from build123d import *

# Parameters (mm, degrees)
SKETCH1_W           = 26
SKETCH1_H           = 50
BOSS_EXTRUDE1_DEPTH = 8
SKETCH2_W           = 26
SKETCH2_H           = 50
BOSS_EXTRUDE2_DEPTH = 8
SKETCH3_W           = 26
SKETCH3_H           = 7
BOSS_EXTRUDE3_DEPTH = 36
SKETCH4_R           = 8
SKETCH4_R_2         = 5
BOSS_EXTRUDE4_DEPTH = 10
FILLET2_R           = 3
SKETCH6_W           = 7
SKETCH6_H           = 17
BOSS_EXTRUDE5_DEPTH = 20
CHAMFER1_SIZE       = 2
CUT_EXTRUDE2_DEPTH  = 0.5
CUT_EXTRUDE3_DEPTH  = 0.5
CUT_EXTRUDE4_REACH  = 90.986
SKETCH11_W          = 26
SKETCH11_H          = 10
CUT_EXTRUDE5_DEPTH  = 3
SKETCH12_W          = 26
SKETCH12_H          = 10
CUT_EXTRUDE6_DEPTH  = 3
CUT_EXTRUDE7_REACH  = 90.986
SKETCH13_R          = 1.5
SKETCH14_W          = 39.670907723
SKETCH14_H          = 70.738486061
CUT_EXTRUDE8_DEPTH  = 8
SKETCH15_W          = 26
SKETCH15_H          = 39.127202372
CUT_EXTRUDE9_DEPTH  = 28.5


with BuildPart() as part:
    # Sketch1 → Boss-Extrude1 (new body)
    with BuildSketch(Plane.XY):
        with Locations((37.264100782, -29)):
            Rectangle(SKETCH1_W, SKETCH1_H)
        with BuildLine():
            Line((39.049457889, -22.265997948), (35.478743675, -22.265997948))
            ThreePointArc((35.478743675, -22.265997948), (34.764100782, -20.515997948), (35.478743675, -18.765997947))
            Line((35.478743675, -18.765997947), (39.049457889, -18.765997947))
            ThreePointArc((39.049457889, -18.765997947), (39.764100782, -20.515997948), (39.049457889, -22.265997948))
        make_face(mode=Mode.SUBTRACT)
    extrude(amount=BOSS_EXTRUDE1_DEPTH)



with BuildPart() as body_2:
    # Sketch2 → Boss-Extrude2 (new body)
    with BuildSketch(Plane(origin=(0, 0, -20), x_dir=(-1, 0, 0), z_dir=(0, 0, -1))):
        with Locations((-37.264100782, -29)):
            Rectangle(SKETCH2_W, SKETCH2_H)
        with BuildLine():
            Line((-39.049457889, -18.765997947), (-35.478743675, -18.765997947))
            ThreePointArc((-35.478743675, -18.765997947), (-34.764100782, -20.515997948), (-35.478743675, -22.265997948))
            Line((-35.478743675, -22.265997948), (-39.049457889, -22.265997948))
            ThreePointArc((-39.049457889, -22.265997948), (-39.764100782, -20.515997948), (-39.049457889, -18.765997947))
        make_face(mode=Mode.SUBTRACT)
    extrude(amount=BOSS_EXTRUDE2_DEPTH)


with BuildPart() as part_1:
    add(part.part)

    add(body_2.part)  # Boss-Extrude3 merges body 2
    # Sketch3 → Boss-Extrude3 (add)
    with BuildSketch(Plane.XY.offset(8)):
        with Locations((37.264100782, -50.5)):
            Rectangle(SKETCH3_W, SKETCH3_H)
    extrude(amount=-BOSS_EXTRUDE3_DEPTH)

    # Sketch4 → Boss-Extrude4 (add)
    with BuildSketch(Plane.XZ.offset(54)):
        with Locations(Location((37.264100782, -10, 0), (0, 0, 90))):
            Circle(SKETCH4_R)
        with Locations(Location((37.264100782, -10, 0), (0, 0, 270))):
            Circle(SKETCH4_R_2, mode=Mode.SUBTRACT)
    extrude(amount=BOSS_EXTRUDE4_DEPTH)

    # Fillet2
    fillet2_edges = [part_1.edges().sort_by_distance(p)[0] for p in [
        (24.264100782, -29, 8),
        (24.264100782, -29, -28),
    ]]
    fillet(fillet2_edges, radius=FILLET2_R)

    # Sketch6 → Boss-Extrude5 (add)
    with BuildSketch(Plane.XY.offset(-20)):
        with Locations((27.764100782, -45.5)):
            Rectangle(SKETCH6_W, SKETCH6_H)
    extrude(amount=BOSS_EXTRUDE5_DEPTH)

    # Chamfer1
    chamfer1_edges = [part_1.edges().sort_by_distance(p)[0] for p in [
        (37.264100782, -54, -18),
    ]]
    chamfer(chamfer1_edges, length=CHAMFER1_SIZE)

    # Sketch7 → Cut-Extrude2 (cut)
    with BuildSketch(Plane(origin=(0, 0, 0), x_dir=(-1, 0, 0), z_dir=(0, 0, -1))):
        Polygon((-50.264100782, -4), (-50.264100782, -47), (-31.264100782, -47), (-31.264100782, -37), (-24.264100782, -37), (-24.264100782, -4), align=None)
    extrude(amount=-CUT_EXTRUDE2_DEPTH, mode=Mode.SUBTRACT)

    # Sketch8 → Cut-Extrude3 (cut)
    with BuildSketch(Plane.XY.offset(-20)):
        Polygon((50.264100782, -47), (50.264100782, -4), (24.264100782, -4), (24.264100782, -37), (31.264100782, -37), (31.264100782, -47), align=None)
    extrude(amount=-CUT_EXTRUDE3_DEPTH, mode=Mode.SUBTRACT)

    # Cut-Extrude4: up to this face of the body (flat: up to its plane)
    cut_extrude4_end = Plane(part_1.part.faces().sort_by_distance((38.785185957, -29.119257779, -28))[0])
    # Sketch10 → Cut-Extrude4 (cut, up to the picked face)
    with BuildSketch(Plane.XY.offset(8), mode=Mode.PRIVATE) as cut_extrude4_sk1:
        with BuildLine():
            Line((50.264100782, -20.515997948), (50.264100782, 2.26582648))
            Line((50.264100782, 2.26582648), (24.264100782, 2.26582648))
            Line((24.264100782, 2.26582648), (24.264100782, -20.515997948))
            ThreePointArc((24.264100782, -20.515997948), (37.264100782, -7.515997948), (50.264100782, -20.515997948))
        make_face()
    cut_extrude4_tool1 = split(extrude(cut_extrude4_sk1.sketch, amount=-CUT_EXTRUDE4_REACH, mode=Mode.PRIVATE), bisect_by=cut_extrude4_end, keep=Keep.BOTH, mode=Mode.PRIVATE)
    add(cut_extrude4_tool1.solids().sort_by(Axis((37.264101, -4.354837, 8), (0, 0, -1)))[0], mode=Mode.SUBTRACT)

    # Sketch11 → Cut-Extrude5 (cut)
    with BuildSketch(Plane.XY.offset(8)):
        with Locations((37.264100782, -49)):
            Rectangle(SKETCH11_W, SKETCH11_H)
    extrude(amount=-CUT_EXTRUDE5_DEPTH, mode=Mode.SUBTRACT)

    # Sketch12 → Cut-Extrude6 (cut)
    with BuildSketch(Plane(origin=(0, 0, -28), x_dir=(-1, 0, 0), z_dir=(0, 0, -1))):
        with Locations((-37.264100782, -49)):
            Rectangle(SKETCH12_W, SKETCH12_H)
    extrude(amount=-CUT_EXTRUDE6_DEPTH, mode=Mode.SUBTRACT)

    # Cut-Extrude7: up to this face of the body (flat: up to its plane)
    cut_extrude7_end = Plane(part_1.part.faces().sort_by_distance((38.560022368, -26.898937337, -28))[0])
    # Sketch13 → Cut-Extrude7 (cut, up to the picked face)
    with BuildSketch(Plane.XY.offset(8), mode=Mode.PRIVATE) as cut_extrude7_sk1:
        with Locations((45.264100782, -50.5)):
            Circle(SKETCH13_R)
    cut_extrude7_tool1 = split(extrude(cut_extrude7_sk1.sketch, amount=-CUT_EXTRUDE7_REACH, mode=Mode.PRIVATE), bisect_by=cut_extrude7_end, keep=Keep.BOTH, mode=Mode.PRIVATE)
    # Sketch13 → Cut-Extrude7 (cut, up to the picked face)
    with BuildSketch(Plane.XY.offset(8), mode=Mode.PRIVATE) as cut_extrude7_sk2:
        with Locations((30.264100782, -50.5)):
            Circle(SKETCH13_R)
    cut_extrude7_tool2 = split(extrude(cut_extrude7_sk2.sketch, amount=-CUT_EXTRUDE7_REACH, mode=Mode.PRIVATE), bisect_by=cut_extrude7_end, keep=Keep.BOTH, mode=Mode.PRIVATE)
    # Sketch13 → Cut-Extrude7 (cut, up to the picked face)
    with BuildSketch(Plane.XY.offset(8), mode=Mode.PRIVATE) as cut_extrude7_sk3:
        with Locations(Location((27.764100782, -40.5, 0), (0, 0, 109.471220634))):
            Circle(SKETCH13_R)
    cut_extrude7_tool3 = split(extrude(cut_extrude7_sk3.sketch, amount=-CUT_EXTRUDE7_REACH, mode=Mode.PRIVATE), bisect_by=cut_extrude7_end, keep=Keep.BOTH, mode=Mode.PRIVATE)
    add(cut_extrude7_tool1.solids().sort_by(Axis((45.264101, -50.5, 8), (0, 0, -1)))[0], mode=Mode.SUBTRACT)
    add(cut_extrude7_tool2.solids().sort_by(Axis((30.264101, -50.5, 8), (0, 0, -1)))[0], mode=Mode.SUBTRACT)
    add(cut_extrude7_tool3.solids().sort_by(Axis((27.764101, -40.5, 8), (0, 0, -1)))[0], mode=Mode.SUBTRACT)

    # Sketch14 → Cut-Extrude8 (cut)
    with BuildSketch(Plane(origin=(0, 0, -28), x_dir=(-1, 0, 0), z_dir=(0, 0, -1))):
        with Locations((-35.76618016, -37.229796089)):
            Rectangle(SKETCH14_W, SKETCH14_H)
    extrude(amount=-CUT_EXTRUDE8_DEPTH, mode=Mode.SUBTRACT)

    # Chamfer2: read off the stored shape, not the designer's step
    # Chamfer2 outline → Chamfer2 (revolve, cut)
    with BuildSketch(Plane(origin=(27.764100782, -40.5, 0), x_dir=(1, 0, 0), z_dir=(0, -1, 0))):
        Polygon((1.5, 8.000002987), (1.5, 7), (2.500002987, 8.000002987), align=None)
    revolve(axis=Axis((27.764100782, -40.5, 0), (0, 0, 1)), mode=Mode.SUBTRACT)

    # Sketch15 → Cut-Extrude9 (cut)
    with BuildSketch(Plane(origin=(0, 0, 0.5), x_dir=(-1, 0, 0), z_dir=(0, 0, -1))):
        with Locations((-37.264100782, -56.563601186)):
            Rectangle(SKETCH15_W, SKETCH15_H)
    extrude(amount=CUT_EXTRUDE9_DEPTH, mode=Mode.SUBTRACT)


solid = part_1.part
Work out the finished part from the listing and answer in its coordinate system (mm). A direction names the side the tool comes from. Round coordinates to 2 decimals unless told otherwise and drop trailing zeros. Write each loop counter-clockwise with the first axis right and the second up, starting at its lowest first coordinate (ties: lowest second). Pieces come first, ordered by that corner, then holes. Notation, with made-up numbers: (-17.75, -1) - (-12.75, -1) arc R22 cw to (-12.75, 26) - close; hole circle Ø4 at (-12, 57). An arc over 180 degrees is marked (long way). Answer in a Markdown table with one row per item. Add a question column.
1. The mould has two halves that part along Y. Classify faces 4 (the conical face through (29.36, -40, 7.17)), 5 (the cylindrical face through (36.98, -7.52, 4.3)), 6 (the flat face through (37, -49, 5)): +Y half, -Y half, draft (parallel to the pull), parting line (faces both ways), or undercut.
2. A cutting plane is placed at C-C, the plane z = 2.5. Determine the outline of the cut face in (x, y).
3. A cutting plane is placed at B-B, the plane y = -50.5. Determine the outline of the cut face in (x, z).
4. For faces 1 (the flat face through (37, -30, 0.5)), 2 (the cylindrical face through (34.764, -20.543, 4.198)), 3 (the flat face through (37, -44, 7)), determine the directions among +Z, -Z, +X, -X, +Y, -Y from which every point of the face is accessible in a straight line to the end or side of a thin tool.
5. A cutting plane is placed at A-A, the plane x = 37.25. Determine the outline of the cut face in (y, z).
6. A cutting plane is placed at D-D, the plane y = -40.5. Determine the outline of the cut face in (x, z), and give its area (3 significant figures).
7. Given pin 1 (1.5 mm diameter, centred on x = 31, z = 6.5, fed in from -Y); pin 2 (8 mm diameter, centred on x = 38, y = -51.5, fed in from +Z); pin 3 (5 mm diameter, centred on x = 27.76, y = -40.5, fed in from -Z); pin 4 (2 mm diameter, centred on y = -18.5, z = 5.5, fed in from +X), each flat-ended and moving along its own axis, determine where each tip first touches the part or whether it passes through.
8. Find the intervals of material crossed by line 1 along Z through (x, y) = (39.25, -49); line 2 along X through (y, z) = (-19.5, 5.5); line 3 along Y through (x, z) = (32.25, 1.75), in increasing order. Write a range as from..to.
Worked out:
| question | item | result |
|---|---|---|
| 1 | face 4 | undercut |
| 1 | face 5 | +Y half |
| 1 | face 6 | draft |
| 2 | outline | (24.26, -54) - (50.26, -54) - (50.26, -20.52) arc R13 ccw to (24.26, -20.52) - close; hole circle Ø3 at (27.76, -40.5); hole circle Ø3 at (30.26, -50.5); hole (35.48, -22.27) - (39.05, -22.27) arc R2.5 ccw to (39.05, -18.77) - (35.48, -18.77) arc R2.5 ccw to start; hole circle Ø3 at (45.26, -50.5) |
| 3 | outline | (24.26, 0.5) - (28.76, 0.5) - (28.76, 5) - (24.26, 5) - close; (31.76, 0.5) - (43.76, 0.5) - (43.76, 5) - (31.76, 5) - close; (46.76, 0.5) - (50.26, 0.5) - (50.26, 5) - (46.76, 5) - close |
| 4 | face 1 | -Z, +X, -X, +Y, -Y |
| 4 | face 2 | +Z, -Z |
| 4 | face 3 | +Z, +X, -X, -Y |
| 5 | outline | (-54, 0.5) - (-22.27, 0.5) - (-22.27, 8) - (-44, 8) - (-44, 5) - (-54, 5) - close; (-18.77, 0.5) - (-7.52, 0.5) - (-7.52, 8) - (-18.77, 8) - close |
| 6 | outline | (24.26, 0.5) - (26.26, 0.5) - (26.26, 7) - (25.7, 7.56) arc R3 ccw to (24.26, 5) - close; (29.26, 0.5) - (50.26, 0.5) - (50.26, 8) - (30.26, 8) - (29.26, 7) - close |
| 6 | area | 170 mm^2 |
| 7 | pin 1 | y = -44 |
| 7 | pin 2 | z = 5 |
| 7 | pin 3 | z = 0.5 |
| 7 | pin 4 | x = 50.22 |
| 8 | line 1 | 0.5..5 |
| 8 | line 2 | 24.31..34.98, 39.55..50.22 |
| 8 | line 3 | -54..-8.52 |
